Autodesk Fusion 360 part; units mm, degrees
sketch "Sketch1" plane through (0, 0, 0) normal (0, 1, 0) x (1, 0, 0)
  line L0 (-0.857, 11.0235) -> (12.013, 11.0235)
  line L1 (14.513, 8.5235) -> (14.513, -4.3565)
  line L2 (12.013, -6.8565) -> (-0.857, -6.8565)
  line L3 (-3.357, -4.3565) -> (-3.357, 8.5235)
  circle A0 centre (-0.672, 8.3235) radius 1.2
  circle A1 centre (11.828, 8.3235) radius 1.2
  line L4 (4.353, 3.1235) -> (6.803, 3.1235)
  line L5 (6.803, 3.1235) -> (6.803, 0.6735)
  line L6 (6.803, 0.6735) -> (4.353, 0.6735)
  line L7 (4.353, 0.6735) -> (4.353, 3.1235)
  circle A2 centre (5.578, -4.4565) radius 0.75
  line L8 (-3.357, -4.4565) -> (14.513, -4.4565)
  circle A3 centre (8.128, -4.4565) radius 0.75
  circle A4 centre (10.678, -4.4565) radius 0.75
  circle A5 centre (3.028, -4.4565) radius 0.75
  circle A6 centre (0.478, -4.4565) radius 0.75
  arc A7 (-0.857, 11.0235) -> (-3.357, 8.5235) centre (-0.857, 8.5235) ccw
  arc A8 (14.513, 8.5235) -> (12.013, 11.0235) centre (12.013, 8.5235) ccw
  arc A9 (12.013, -6.8565) -> (14.513, -4.3565) centre (12.013, -4.3565) ccw
  arc A10 (-3.357, -4.3565) -> (-0.857, -6.8565) centre (-0.857, -4.3565) ccw
  line L9 (5.578, 11.0235) -> (5.578, -6.8565)
  line L10 (-0.672, 8.3235) -> (11.828, 8.3235)
  dimension "d1" = 2.4
  dimension "d4" = 17.88
  dimension "d5" = 2.7
  dimension "d6" = 2.7
  dimension "d7" = 2.45
  dimension "d8" = 2.45
  dimension "d12" = 1.5
  dimension "d13" = 2.4
  dimension "d18" = 2.55
  dimension "d19" = 2.55
  dimension "d20" = 2.55
  dimension "d21" = 2.55
  dimension "d22" = 2.5
  dimension "d27" = 5.2
  dimension "d51" = 12.5
  dimension "d52" = 17.87
extrude "Extrude1" add sketch "Sketch1" along normal blind 1.65 contours L0 L3 L4 L6 L7 A2 L8 A5 A6 A7 A10 L9 | L0 L1 L4 L5 L6 A2 L8 A3 A4 A8 A9 L9 | L2 A2 L8 A5 A6 A10 L9 | L2 A2 L8 A3 A4 A9 L9
extrude "Extrude2" add sketch "Sketch1" along normal blind 2.65 contours L4 L6 L7 L9 | L4 L5 L6 L9
sketch "Sketch2" plane through (0, 1.65, 0) normal (0, 1, 0) x (-1, 0, 0)
  circle A0 centre (-5.578, 4.4565) radius 0.75
  circle A1 centre (-0.478, 4.4565) radius 0.75
  circle A2 centre (0.672, -8.3235) radius 1.2
  circle A3 centre (-10.678, 4.4565) radius 0.75
  circle A4 centre (-8.128, 4.4565) radius 0.75
  line L0 (-6.803, -0.6735) -> (-4.353, -0.6735)
  line L1 (-4.353, -0.6735) -> (-4.353, -3.1235)
  line L2 (-4.353, -3.1235) -> (-6.803, -3.1235)
  line L3 (-6.803, -3.1235) -> (-6.803, -0.6735)
  circle A5 centre (-3.028, 4.4565) radius 0.75
  circle A6 centre (-11.828, -8.3235) radius 1.2
  arc A7 (0.857, -11.0235) -> (3.357, -8.5235) centre (0.857, -8.5235) ccw
  line L4 (3.357, -8.5235) -> (3.357, 4.3565)
  arc A8 (3.357, 4.3565) -> (0.857, 6.8565) centre (0.857, 4.3565) ccw
  line L5 (0.857, 6.8565) -> (-12.013, 6.8565)
  arc A9 (-12.013, 6.8565) -> (-14.513, 4.3565) centre (-12.013, 4.3565) ccw
  line L6 (-14.513, 4.3565) -> (-14.513, -8.5235)
  arc A10 (-14.513, -8.5235) -> (-12.013, -11.0235) centre (-12.013, -8.5235) ccw
  line L7 (-12.013, -11.0235) -> (0.857, -11.0235)
  line L8 (1.8732, -6.733) -> (-2, -6.733)
  line L9 (-2, -6.733) -> (-2, -5)
  line L10 (-2, -5) -> (1.8732, -5)
  line L11 (1.8732, -5) -> (1.8732, -6.733)
  line L12 (1.2394, -5) -> (-1.5006, -5)
  line L13 (-1.5006, -5) -> (-1.5006, 0.1577)
  line L14 (-1.5006, 0.1577) -> (1.2394, 0.1577)
  line L15 (1.2394, 0.1577) -> (1.2394, -5)
  line L16 (1.955, 0.1577) -> (-2.1549, 0.1577)
  line L17 (-2.1549, 0.1577) -> (-2.1549, 2.2229)
  line L18 (-2.1549, 2.2229) -> (1.955, 2.2229)
  line L19 (1.955, 2.2229) -> (1.955, 0.1577)
  line L20 (-3.6884, -0.224) -> (-8.2686, -0.224)
  line L21 (-8.2686, -0.224) -> (-8.2686, 1.731)
  line L22 (-8.2686, 1.731) -> (-3.6884, 1.731)
  line L23 (-3.6884, 1.731) -> (-3.6884, -0.224)
  line L24 (-3.4431, -3.9317) -> (-7.7984, -3.9317)
  line L25 (-7.7984, -3.9317) -> (-7.7984, -6.8557)
  line L26 (-7.7984, -6.8557) -> (-3.4431, -6.8557)
  line L27 (-3.4431, -6.8557) -> (-3.4431, -3.9317)
  line L28 (-9, -6) -> (-13.176, -6)
  line L29 (-13.176, -6) -> (-13.176, -2.5209)
  line L30 (-13.176, -2.5209) -> (-9, -2.5209)
  line L31 (-9, -2.5209) -> (-9, -6)
  line L32 (-8.6776, -1.4781) -> (-13.176, -1.4781)
  line L33 (-13.176, -1.4781) -> (-13.176, 2.2433)
  line L34 (-13.176, 2.2433) -> (-8.6776, 2.2433)
  line L35 (-8.6776, 2.2433) -> (-8.6776, -1.4781)
extrude "Extrude3" add sketch "Sketch2" along normal blind 1.2 contours L8 L9 L10 L11 L12 | L14 L16 L17 L18 L19
extrude "Extrude4" add sketch "Sketch2" along normal blind 0.97 contours L24 L25 L26 L27 | L32 L33 L34 L35
extrude "Extrude5" add sketch "Sketch2" along normal blind 0.5 contours L28 L29 L30 L31
extrude "Extrude6" add sketch "Sketch2" along normal blind 1.15 contours L10 L12 L13 L14 L15 L16
extrude "Extrude7" add sketch "Sketch2" along normal blind 0.81 contours L20 L21 L22 L23
sketch "Sketch3" plane through (0, 2.65, 0) normal (0, 1, 0) x (-1, 0, 0)
  line L0 (-4.353, -0.6735) -> (-6.803, -0.6735)
  line L1 (-6.803, -0.6735) -> (-6.803, -3.1235)
  line L2 (-6.803, -3.1235) -> (-4.353, -3.1235)
  line L3 (-4.353, -3.1235) -> (-4.353, -0.6735)
  circle A0 centre (-5.578, -1.8985) radius 0.58
  line L4 (-5.578, -3.1235) -> (-5.578, -0.6735)
  line L5 (-5.578, -1.8985) -> (-4.9008, -2.5757)
  line L6 (-5.578, -1.8985) -> (-4.4704, -1.8985) construction
  line L7 (-4.9008, -2.5757) -> (-5.0253, -2.7001)
  line L8 (-5.0253, -2.7001) -> (-5.3117, -2.4137)
  line L9 (-4.9008, -2.5757) -> (-4.7764, -2.4512)
  line L10 (-4.7764, -2.4512) -> (-5.0628, -2.1648)
  dimension "d44" = 1.16
  dimension "d45" = 45
extrude "Extrude8" cut sketch "Sketch3" against normal blind 0.01 contours A0 L4 | A0 L4 L5 | A0 L4 L5 | A0 L5 L9 L10 | A0 L5 L7 L8
equation "d5 = 1.5 mm + ( ( 2.4 / 2 ) * 1 mm )"
equation "d27 = 4.0 mm + ( ( 2.4 / 2 ) * 1 mm )"
equation "d34 = 2.85 mm - 1.65 mm"
equation "d36 = 2.62 mm - 1.65 mm"
equation "d38 = 2.15 mm - 1.65 mm"
equation "d40 = 2.8 mm - 1.65 mm"
equation "d42 = 2.46 mm - 1.65 mm"
Geometry: final body of the model. Coordinates: model frame, mm. A direction names the side the tool comes from. Round coordinates to 2 decimals unless told otherwise and drop trailing zeros. Loops run counter-clockwise (first coordinate to the right, second up) from the corner with the lowest first, then second, coordinate; pieces in that order, holes last. Notation, with made-up numbers: (-8.5, -19.75) -> (34.5, -19.75) arc R19 ccw to (34.5, -9.75) -> close; hole circle Ø1 at (-21, 70). An arc over 180 degrees is marked (long way). Use one line per item in the form item = value. Start each with the question number.
1) Access query for faces 1 (the flat face through (2, 2, -6)), 2 (the flat face through (1.501, 2, -2)), 3 (the flat face through (11, 2.15, -4)), 4 (the flat face through (11, 2.62, 0)), 5 (the flat face through (3.688, 2, 1)). Directions: +Z, -Z, +X, -X, +Y, -Y. A direction counts if a zero-diameter tool reaches every point of the face in a straight line with its end or side. Return the directions, or none.
2) First-contact query: P1, Ø0.8, axis at x = 6, y = 2.5, coming from the +Z side; P2, Ø5, axis at x = 12.5, z = 3.5, coming from the -Y side; P3, Ø0.5, axis at y = 2, z = -6, coming from the -X side; P4, Ø2, axis at x = 6, z = -2, coming from the +Y side. Flat tips, straight axial feed; report the tip coordinate or a pass-through.
3) Line query: L1, parallel to X at y = 2.4, z = 1 (3 decimals); L2, parallel to X at y = 1.85, z = -5.75; L3, parallel to Z at x = 5, y = 2.4. Output: solid intervals per line, ascending.
4) Draft query along X for faces 6 (the flat face through (-1.239, 2, -2)), 7 (the flat face through (6, 2.46, 1)), 8 (the flat face through (0, 2.85, 1)). Return one class per face: released by +X, released by -X, zero draft, split by the parting line, or undercut.
5) Section A-A on z = -5.5. Output: boundary loops of the cut face in (x, y).
6) Section B-B on x = 9.5. Output: boundary loops of the cut face in (y, z), then the cut area to 3 significant figures.
7) Section D-D on y = 0.7. Output: boundary loops of the cut face in (x, z), then the cut area to 3 significant figures.
8) Section C-C on x = 0.25. Output: boundary loops of the cut face in (y, z).
Response:
q1.face_1 = -Z, +Y
q1.face_2 = +Y
q1.face_3 = -Z, +X, +Y
q1.face_4 = +Z, -Z, +X, +Y
q1.face_5 = +Z, +Y
q2.P1 = 1.73
q2.P2 = 0
q2.P3 = -1.87
q2.P4 = 2.65
q3.L1 = -1.955 to 2.155, 3.688 to 8.269, 8.678 to 13.176
q3.L2 = -1.87 to 2, 3.44 to 7.8, 9 to 13.18
q3.L3 = -6.86 to -3.93, -3.12 to -0.67, -0.22 to 1.73
q4.face_6 = released by -X
q4.face_7 = undercut
q4.face_8 = zero draft
q5.outline = (-3.36, 0) -> (14.51, 0) -> (14.51, 1.65) -> (13.18, 1.65) -> (13.18, 2.15) -> (9, 2.15) -> (9, 1.65) -> (7.8, 1.65) -> (7.8, 2.62) -> (3.44, 2.62) -> (3.44, 1.65) -> (2, 1.65) -> (2, 2.85) -> (-1.87, 2.85) -> (-1.87, 1.65) -> (-3.36, 1.65) -> close
q6.outline = (0, -11.02) -> (1.65, -11.02) -> (1.65, -6) -> (2.15, -6) -> (2.15, -2.52) -> (1.65, -2.52) -> (1.65, -1.48) -> (2.62, -1.48) -> (2.62, 2.24) -> (1.65, 2.24) -> (1.65, 6.86) -> (0, 6.86) -> close
q6.area = 34.9 mm^2
q7.outline = (-3.36, -8.52) arc R2.5 ccw to (-0.86, -11.02) -> (12.01, -11.02) arc R2.5 ccw to (14.51, -8.52) -> (14.51, 4.36) arc R2.5 ccw to (12.01, 6.86) -> (-0.86, 6.86) arc R2.5 ccw to (-3.36, 4.36) -> close; hole circle Ø2.4 at (-0.67, -8.32); hole circle Ø1.5 at (0.48, 4.46); hole circle Ø1.5 at (3.03, 4.46); hole circle Ø1.5 at (5.58, 4.46); hole circle Ø1.5 at (8.13, 4.46); hole circle Ø1.5 at (10.68, 4.46); hole circle Ø2.4 at (11.83, -8.32)
q7.area = 296 mm^2
q8.outline = (0, -11.02) -> (1.65, -11.02) -> (1.65, -9.09) -> (0, -9.09) -> close; (0, -7.56) -> (1.65, -7.56) -> (1.65, -6.73) -> (2.85, -6.73) -> (2.85, -5) -> (2.8, -5) -> (2.8, 0.16) -> (2.85, 0.16) -> (2.85, 2.22) -> (1.65, 2.22) -> (1.65, 3.74) -> (0, 3.74) -> close; (0, 5.17) -> (1.65, 5.17) -> (1.65, 6.86) -> (0, 6.86) -> close
